```python
from build123d import *

# Parameters (mm, degrees)
F0_R     = 5.25
F0_W     = 0.75
F0_H     = 8
F1_DEPTH = 9


# Not quite as in the source:
# - a feature names something its author has since deleted; it is built from what else it names


with BuildPart() as f1:
    # F0 (on Front) → F1 (new body)
    with BuildSketch(Plane.XZ):
        Polygon((29, 0), (21, 0), (21, -8), (21, -109.6278309861), (21, -116.8163269758), (161, -53.9573058486), align=None)
        with Locations((31, -94.8660687473)):
            Circle(F0_R, mode=Mode.SUBTRACT)
        with Locations((31, -14.8660687473)):
            Circle(F0_R, mode=Mode.SUBTRACT)
        Polygon((43.1111576917, -75.528110744), (43.1111576917, -21.972979021), (61.8685626933, -29.6403959801), (71.7187130056, -33.6668169881), (86.6322777796, -39.7629971078), (95.6788662869, -43.460948191), (116.6788079217, -52.0450411727), (86.5560721122, -65.7548940175), (73.5966112911, -71.6531730426), (52.2128066716, -81.3856494169), (43.1111576917, -85.528110744), align=None, mode=Mode.SUBTRACT)
        with Locations((133.4695076596, -54.8660687473)):
            Circle(F0_R, mode=Mode.SUBTRACT)
        Polygon((71.7187130056, -33.6668169881), (61.8685626933, -29.6403959801), (43.1111576917, -75.528110744), (43.1111576917, -85.528110744), (52.2128066716, -81.3856494169), align=None)
        Polygon((21, -8), (21, 0), (-8, 0), (-8, -20), (0, -20), (0, -12), (0, -8), align=None)
        with Locations((0.375, -16)):
            Rectangle(F0_W, F0_H)
        Polygon((95.6788662869, -43.460948191), (86.6322777796, -39.7629971078), (73.5966112911, -71.6531730426), (86.5560721122, -65.7548940175), (86.6322777796, -65.5923289964), (92.8699112608, -50.3327157415), align=None)
    extrude(amount=F1_DEPTH)


solid = f1.part
```
Check sheet for the modelled part. Datum: model origin and axes. Units: mm. A direction names the side the tool comes from. Give positions to 0.01 mm unless a question says otherwise; leave off trailing zeros. Order: outer loops, then holes, each group sorted by start corner. A loop starts at its lowest first (then second) coordinate and runs counter-clockwise, first axis right, second up. Notation, with made-up numbers: (61, -36.5) -> (80, -36.5) arc R18 ccw to (80, -29.5) -> close; hole circle Ø2 at (81.25, 36.25). An arc over 180 degrees is marked (long way). Use CSV: the item, a comma, the result in double quotes. Start each with the question number.
1) Go/stop test with flat-tipped pins: P1, Ø2.5, axis at y = -6, z = -58, coming from the +X side; P2, Ø2.5, axis at y = -3, z = -14.5, coming from the +X side; P3, Ø4, axis at x = 84.5, y = -2.5, coming from the -Z side. Record where each tip stops, or that it passes through.
2) Sectioned sample at A-A, the plane z = -70. Record the boundary of the cut face in (x, y).
3) Set-up check for faces 1 (the face through (90.02, -4.437, -85.827)), 2 (the face through (80.2, -4.4, -55.5)), 3 (the face through (-4, -4, -20)): record each of +Z, -Z, +X, -X, +Y, -Y from which the full face is reachable in a straight line by a thin tool's end or side.
4) Sectioned sample at D-D, the plane z = -46. Record the boundary of the cut face in (x, y).
5) Sectioned sample at B-B, the plane x = 31. Record the boundary of the cut face in (y, z).
6) Sectioned sample at C-C, the plane y = -2.25. Record the boundary of the cut face in (x, z).
7) Material ranges on line 1 (Z direction, x = 31, y = -4); line 2 (Z direction, x = 55, y = -3); line 3 (X direction, y = -1, z = -47), recorded low to high. Write a range as from..to.
Recorded:
1,P1,"x = 154.78"
1,P2,"x = 67.53"
1,P3,"z = -89.2"
2,outline,"(21, -9) -> (43.11, -9) -> (43.11, 0) -> (21, 0) -> close; (45.37, -9) -> (56.87, -9) -> (56.87, 0) -> (45.37, 0) -> close; (74.27, -9) -> (125.27, -9) -> (125.27, 0) -> (74.27, 0) -> close"
3,face 1,"-Z, +X, +Y, -Y"
3,face 2,"+Y, -Y"
3,face 3,"-Z, -X, +Y, -Y"
4,outline,"(21, -9) -> (43.11, -9) -> (43.11, 0) -> (21, 0) -> close; (55.18, -9) -> (66.68, -9) -> (66.68, 0) -> (55.18, 0) -> close; (84.08, -9) -> (94.64, -9) -> (94.64, 0) -> (84.08, 0) -> close; (101.89, -9) -> (141.53, -9) -> (141.53, 0) -> (101.89, 0) -> close"
5,outline,"(-9, -112.33) -> (0, -112.33) -> (0, -100.12) -> (-9, -100.12) -> close; (-9, -89.62) -> (0, -89.62) -> (0, -20.12) -> (-9, -20.12) -> close; (-9, -9.62) -> (0, -9.62) -> (0, -0.82) -> (-9, -0.82) -> close"
6,outline,"(-8, -20) -> (0.75, -20) -> (0.75, -12) -> (0, -12) -> (0, -8) -> (21, -8) -> (21, -116.82) -> (161, -53.96) -> (29, 0) -> (-8, 0) -> close; hole circle Ø10.5 at (31, -94.87); hole circle Ø10.5 at (31, -14.87); hole (43.11, -75.53) -> (61.87, -29.64) -> (43.11, -21.97) -> close; hole (52.21, -81.39) -> (73.6, -71.65) -> (86.63, -39.76) -> (71.72, -33.67) -> close; hole (86.56, -65.75) -> (116.68, -52.05) -> (95.68, -43.46) -> (86.63, -65.59) -> close; hole circle Ø10.5 at (133.47, -54.87)"
7,line 1,"-112.33..-100.12, -89.62..-20.12, -9.62..-0.82"
7,line 2,"-101.55..-80.12, -74.57..-46.44, -26.83..-10.63"
7,line 3,"21..43.11, 54.77..66.27, 83.67..94.23, 104.34..143.98"
